```python
from build123d import *

# Parameters (mm, degrees)
SKETCH_8_W                = 220
SKETCH_8_H                = 120
EXTRUDE_6_DEPTH           = 3
SKETCH_10_W               = 10
SKETCH_10_H               = 120
EXTRUDE_7_DEPTH           = 27
CUT_EXTRUDE_1_DEPTH       = 129.175660716
CUT_EXTRUDE_1_DEPTH_BACK  = 129.175660716
SKETCH_9_R                = 2.05
SKETCH_11_R               = 3.6
CUT_EXTRUDE_2_DEPTH       = 22
CUT_EXTRUDE_4_DEPTH       = 129.175660716
CUT_EXTRUDE_4_DEPTH_BACK  = 129.175660716
SKETCH_13_W               = 40
SKETCH_13_H               = 18.5
SKETCH_14_W               = 140
SKETCH_14_H               = 44
CUT_EXTRUDE_7_DEPTH       = 1
SKETCH_15_W               = 15
SKETCH_15_H               = 80
SKETCH_15_H_2             = 40
SKETCH_15_W_2             = 30
SKETCH_15_H_3             = 16
CUT_EXTRUDE_8_DEPTH       = 129.840987267
SKETCH_9_5_R              = 2
CUT_EXTRUDE_9_DEPTH       = 129.175660716
CUT_EXTRUDE_13_DEPTH      = 27
SKETCH_20_W               = 135
SKETCH_20_H               = 8
EXTRUDE_8_DEPTH           = 2
FILLET_1_R                = 3
FILLET_2_R                = 2
CUT_EXTRUDE_14_DEPTH      = 129.175660716
CUT_EXTRUDE_14_DEPTH_BACK = 129.175660716


with BuildPart() as part:
    # Sketch 8 → Extrude 6 (new body)
    with BuildSketch(Plane(origin=(0, 0, 0), x_dir=(1, 0, 0), z_dir=(0, 1, 0))):
        Rectangle(SKETCH_8_W, SKETCH_8_H)
    extrude(amount=EXTRUDE_6_DEPTH)

    # Sketch 10 → Extrude 7 (add)
    with BuildSketch(Plane.XZ):
        with Locations((-105, 0)):
            Rectangle(SKETCH_10_W, SKETCH_10_H)
        with Locations((105, 0)):
            Rectangle(SKETCH_10_W, SKETCH_10_H)
    extrude(amount=EXTRUDE_7_DEPTH)

    # Sketch 9 → Cut-Extrude 1 (cut, two sides: drawn at the far end of the back side and taken through both)
    with BuildSketch(Plane(origin=(0, 0, 0), x_dir=(1, 0, 0), z_dir=(0, 1, 0)).offset(-CUT_EXTRUDE_1_DEPTH_BACK)):
        with Locations(Location((104.5, 54.5, 0), (0, 0, 270))):
            Circle(SKETCH_9_R)
        with Locations(Location((-104.5, 54.5, 0), (0, 0, 90))):
            Circle(SKETCH_9_R)
        with Locations(Location((-104.5, -54.5, 0), (0, 0, 270))):
            Circle(SKETCH_9_R)
        with Locations(Location((104.5, -54.5, 0), (0, 0, 90))):
            Circle(SKETCH_9_R)
    extrude(amount=CUT_EXTRUDE_1_DEPTH + CUT_EXTRUDE_1_DEPTH_BACK, mode=Mode.SUBTRACT)

    # Sketch 11 → Cut-Extrude 2 (cut)
    with BuildSketch(Plane(origin=(0, 3, 0), x_dir=(1, 0, 0), z_dir=(0, 1, 0))):
        with Locations(Location((-104.497380754, 54.5, 0), (0, 0, 270))):
            Circle(SKETCH_11_R)
        with Locations(Location((-104.497380754, -54.5, 0), (0, 0, 90))):
            Circle(SKETCH_11_R)
        with Locations(Location((104.5, -54.5, 0), (0, 0, 270))):
            Circle(SKETCH_11_R)
        with Locations(Location((104.5, 54.5, 0), (0, 0, 90))):
            Circle(SKETCH_11_R)
    extrude(amount=-CUT_EXTRUDE_2_DEPTH, mode=Mode.SUBTRACT)

    # Sketch 13 → Cut-Extrude 4 (cut, two sides: drawn at the far end of the back side and taken through both)
    with BuildSketch(Plane(origin=(0, 0, 0), x_dir=(0, 0, -1), z_dir=(1, 0, 0)).offset(-CUT_EXTRUDE_4_DEPTH_BACK)):
        with Locations((-25, -12.75)):
            Rectangle(SKETCH_13_W, SKETCH_13_H)
        with Locations((25, -12.75)):
            Rectangle(SKETCH_13_W, SKETCH_13_H)
    extrude(amount=CUT_EXTRUDE_4_DEPTH + CUT_EXTRUDE_4_DEPTH_BACK, mode=Mode.SUBTRACT)

    # Sketch 14 → Cut-Extrude 7 (cut)
    with BuildSketch(Plane(origin=(0, 3, 0), x_dir=(1, 0, 0), z_dir=(0, 1, 0))):
        Rectangle(SKETCH_14_W, SKETCH_14_H)
    extrude(amount=-CUT_EXTRUDE_7_DEPTH, mode=Mode.SUBTRACT)

    # Sketch 15 → Cut-Extrude 8 (cut, through all)
    with BuildSketch(Plane(origin=(0, 3, 0), x_dir=(1, 0, 0), z_dir=(0, 1, 0))):
        with Locations((-92.5, 0)):
            Rectangle(SKETCH_15_W, SKETCH_15_H)
        with Locations((92.5, 25)):
            Rectangle(SKETCH_15_W, SKETCH_15_H_2)
        Polygon((-44.702941459, -12), (44.702941459, -12), (0, -3.059411708), align=None)
        Polygon((-60, -8.940588292), (-60, 8.940588292), (-15.297058541, 0), align=None)
        Polygon((-44.702941459, 12), (44.702941459, 12), (0, 3.059411708), align=None)
        Polygon((60, -8.940588292), (60, 8.940588292), (15.297058541, 0), align=None)
        with Locations((0, -43)):
            Rectangle(SKETCH_15_W_2, SKETCH_15_H_3)
        with Locations((0, 43)):
            Rectangle(SKETCH_15_W_2, SKETCH_15_H_3)
        with Locations((92.5, -25)):
            Rectangle(SKETCH_15_W, SKETCH_15_H_2)
    extrude(amount=-CUT_EXTRUDE_8_DEPTH, mode=Mode.SUBTRACT)

    # Sketch 9_5 → Cut-Extrude 9 (cut, through all)
    with BuildSketch(Plane(origin=(0, 0, 0), x_dir=(1, 0, 0), z_dir=(0, 1, 0))):
        with Locations(Location((30, 28, 0), (0, 0, 270))):
            Circle(SKETCH_9_5_R)
        with Locations(Location((-30, 28, 0), (0, 0, 90))):
            Circle(SKETCH_9_5_R)
        with Locations(Location((30, -28, 0), (0, 0, 90))):
            Circle(SKETCH_9_5_R)
        with Locations(Location((-30, -28, 0), (0, 0, 270))):
            Circle(SKETCH_9_5_R)
    extrude(amount=CUT_EXTRUDE_9_DEPTH, mode=Mode.SUBTRACT)

    # Sketch 19 → Cut-Extrude 13 (cut)
    with BuildSketch(Plane.XZ.offset(27)):
        with BuildLine():
            Line((-100, 54.5), (-100, -54.5))
            ThreePointArc((-100, -54.5), (-101.318019485, -51.318019485), (-104.5, -50))
            Line((-104.5, -50), (-107, -50))
            Line((-107, -50), (-107, 50))
            Line((-107, 50), (-104.5, 50))
            ThreePointArc((-104.5, 50), (-101.318019485, 51.318019485), (-100, 54.5))
        make_face()
        with BuildLine():
            Line((100, 54.5), (100, -54.5))
            ThreePointArc((100, -54.5), (101.318019485, -51.318019485), (104.5, -50))
            Line((104.5, -50), (107, -50))
            Line((107, -50), (107, 50))
            Line((107, 50), (104.5, 50))
            ThreePointArc((104.5, 50), (101.318019485, 51.318019485), (100, 54.5))
        make_face()
    extrude(amount=-CUT_EXTRUDE_13_DEPTH, mode=Mode.SUBTRACT)

    # Sketch 20 → Extrude 8 (add)
    with BuildSketch(Plane.XZ):
        with Locations((0, 56)):
            Rectangle(SKETCH_20_W, SKETCH_20_H)
        with Locations((0, -56)):
            Rectangle(SKETCH_20_W, SKETCH_20_H)
        Polygon((-59, 32.5), (-39, 32.5), (-39, 29.5), (-54, 29.5), (-54, 25), (-59, 25), align=None)
        Polygon((54, 29.5), (39, 29.5), (39, 32.5), (59, 32.5), (59, 25), (54, 25), align=None)
        Polygon((59, -32.5), (39, -32.5), (39, -29.5), (54, -29.5), (54, -25), (59, -25), align=None)
        Polygon((-54, -29.5), (-39, -29.5), (-39, -32.5), (-59, -32.5), (-59, -25), (-54, -25), align=None)
    extrude(amount=EXTRUDE_8_DEPTH)

    # Fillet 1
    fillet_1_edges = [part.edges().sort_by_distance(p)[0] for p in [
        (-110, -12, -60),
        (110, -12, -60),
        (110, -12, 60),
        (-110, -12, 60),
    ]]
    fillet(fillet_1_edges, radius=FILLET_1_R)

    # Fillet 2
    fillet_2_edges = [part.edges().sort_by_distance(p)[0] for p in [
        (-108.5, -3.5, 45),
        (-108.5, -3.5, 5),
        (-108.5, -22, 5),
        (-108.5, -3.5, -5),
        (-108.5, -3.5, -45),
        (-108.5, -22, -45),
        (-108.5, -22, -5),
        (-85, 1.5, -40),
        (-100, 1.5, -40),
        (-85, 1.5, 40),
        (-100, 1.5, 40),
        (-15, 1.5, 51),
        (-15, 1.5, 35),
        (15, 1.5, 35),
        (15, 1.5, 51),
        (100, 1.5, 45),
        (85, 1.5, 5),
        (100, 1.5, 5),
        (15.297058541, 1, 0),
        (60, 1, -8.940588292),
        (60, 1, 8.940588292),
        (0, 1, -3.059411708),
        (-44.702941459, 1, -12),
        (44.702941459, 1, -12),
        (85, 1.5, -5),
        (100, 1.5, -5),
        (85, 1.5, -45),
        (100, 1.5, -45),
        (-15.297058541, 1, 0),
        (-60, 1, 8.940588292),
        (-60, 1, -8.940588292),
        (-15, 1.5, -35),
        (-15, 1.5, -51),
        (15, 1.5, -51),
        (15, 1.5, -35),
        (-44.702941459, 1, 12),
        (0, 1, 3.059411708),
        (44.702941459, 1, 12),
        (108.5, -3.5, 45),
        (108.5, -22, 45),
        (108.5, -3.5, 5),
        (108.5, -22, 5),
        (108.5, -3.5, -45),
        (108.5, -3.5, -5),
        (108.5, -22, -45),
        (108.5, -22, -5),
        (-107, 0, 0),
        (107, 0, 0),
        (-108.5, -22, 45),
    ]]
    fillet(fillet_2_edges, radius=FILLET_2_R)

    # Sketch 21 → Cut-Extrude 14 (cut, two sides: drawn at the far end of the back side and taken through both)
    with BuildSketch(Plane.XY.offset(-CUT_EXTRUDE_14_DEPTH_BACK)):
        Polygon((-35, 3), (-35, 1), (35, 1), (35, -27), (-110, -27), (-110, 3), align=None)
    extrude(amount=CUT_EXTRUDE_14_DEPTH + CUT_EXTRUDE_14_DEPTH_BACK, mode=Mode.SUBTRACT)


solid = part.part
```
Model file for the job. Use its own axes, mm. A direction names the side the tool comes from. Coordinates: 2 decimals unless noted, no trailing zeros. Write each loop counter-clockwise with the first axis right and the second up, starting at its lowest first coordinate (ties: lowest second). Pieces come first, ordered by that corner, then holes. Notation, with made-up numbers: (54.5, 3) - (76.5, 3) arc R26 ccw to (76.5, 22) - close; hole circle Ø7 at (13, 6.25). An arc over 180 degrees is marked (long way). One line per item, written item: value. Start each with the question number.
1. Slice it at A-A (z = -41). Write the cut outline in (x, y).
2. Mould opens along X. For faces 1 (the flat face through (35, 0.2, -38.6)), 2 (the flat face through (57, -1, 60)), 3 (the flat face through (44.74, 1.01, 5.89)) say: released by +X, released by -X, zero draft, split by the parting line, or undercut.
3. Slice it at D-D (x = -21). Write the cut outline in (y, z).
4. Flat gauge pins, fed straight in: pin 1 (12 mm diameter, centred on x = -3, z = -2.5, fed in from -Y); pin 2 (6.5 mm diameter, centred on x = 46, z = 57.5, fed in from -Y); pin 3 (2 mm diameter, centred on x = 65, z = -10.5, fed in from -Y). Where does each tip first touch, or does it go through?
5. Tool access for faces 4 (the flat face through (-12.473, 1.507, -5.554)), 5 (the flat face through (108, -22, 25)), 6 (the flat face through (51, -2, -56)): list every direction of +Z, -Z, +X, -X, +Y, -Y with a clear straight run to the whole face (end or side of a thin tool).
6. Probe line 1 (Z direction, x = 104.5, y = -23.25); line 2 (Z direction, x = 14.5, y = 1.5); line 3 (X direction, y = -24.5, z = 54.5). List the from-to ranges inside material, lowest first. Write a range as from..to.
7. Slice it at C-C (x = 43). Write the cut outline in (y, z).
8. Slice it at B-B (y = -9.25). Write the cut outline in (x, z).
Answers below:
1. outline: (-35, 1) - (-15, 1) - (-15, 3) - (-35, 3) - close; (15, 1) - (35, 1) - (35, 0) - (85, 0) - (85, 3) - (15, 3) - close; (100, 0) - (105, 0) arc R2 cw to (107, -2) - (107, -3.5) - (110, -3.5) - (110, 3) - (100, 3) - close; (107, -27) - (110, -27) - (110, -22) - (107, -22) - close
2. face 1: released by -X
2. face 2: zero draft
2. face 3: undercut
3. outline: (1, -60) - (3, -60) - (3, -22) - (2, -22) - (2, -12) - (1, -12) - close; (1, -7.26) - (2, -7.26) - (2, 7.26) - (1, 7.26) - close; (1, 12) - (2, 12) - (2, 22) - (3, 22) - (3, 60) - (1, 60) - close
4. pin 1: stops at y = 1
4. pin 2: stops at y = -2
4. pin 3: stops at y = 0
5. face 4: +Y, -Y
5. face 5: +X, -X
5. face 6: +Z, -Z, -X, -Y
6. line 1: z = -60..-56.55, -52.45..-50, 50..52.45, 56.55..60
6. line 2: z = -60..-50.32, -35.68..-12, -5.96..5.96, 12..35.68, 50.32..60
6. line 3: x = 100..102.45, 106.55..110
7. outline: (-2, -60) - (3, -60) - (3, -22) - (2, -22) - (2, -5.54) - (0, -5.54) - (0, -29.5) - (-2, -29.5) - (-2, -32.5) - (0, -32.5) - (0, -52) - (-2, -52) - close; (-2, 29.5) - (0, 29.5) - (0, 5.54) - (2, 5.54) - (2, 22) - (3, 22) - (3, 60) - (-2, 60) - (-2, 52) - (0, 52) - (0, 32.5) - (-2, 32.5) - close
8. outline: (100, -60) - (107, -60) arc R3 ccw to (110, -57) - (110, -45) - (107, -45) - (107, -50) - (104.5, -50) arc R4.5 ccw to (100, -54.5) - close; (100, 54.5) arc R4.5 ccw to (104.5, 50) - (107, 50) - (107, 45) - (110, 45) - (110, 57) arc R3 ccw to (107, 60) - (100, 60) - close; (107, -5) - (110, -5) - (110, 5) - (107, 5) - close; hole circle Ø7.2 at (104.5, -54.5); hole circle Ø7.2 at (104.5, 54.5)
